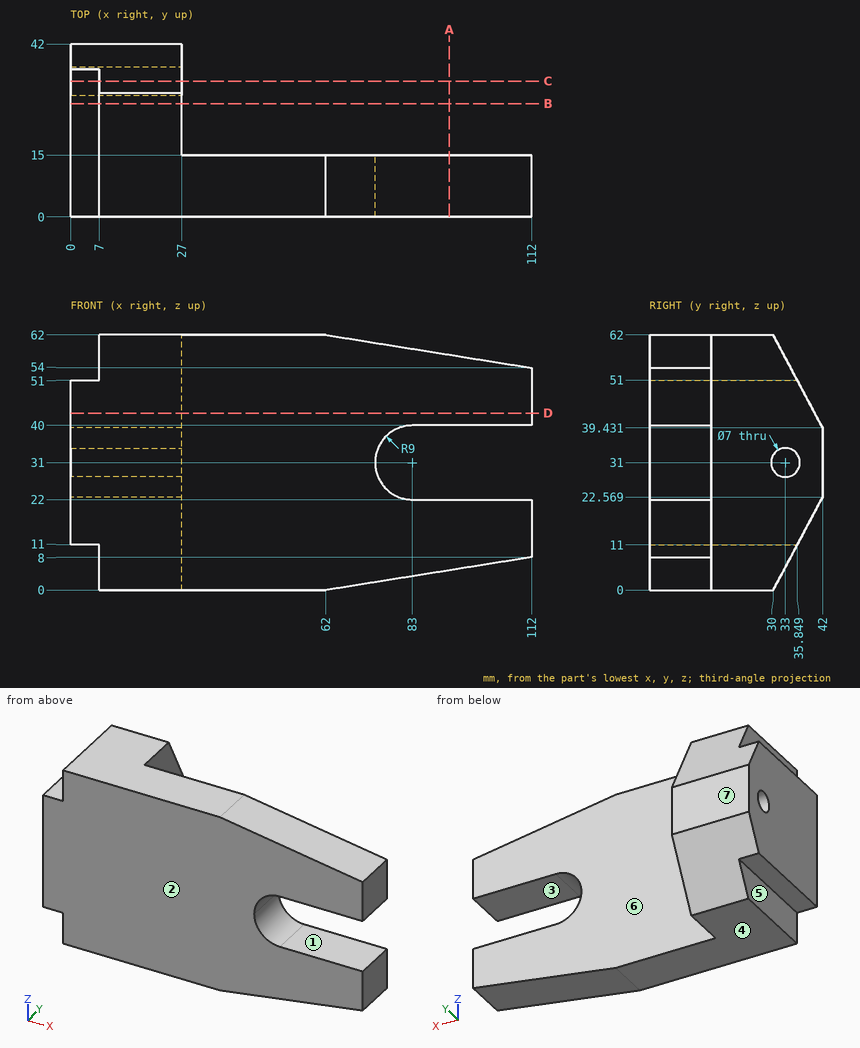
Answer from the drawing. Dimensions are ordinates in mm from the lowest x, y and z of the part. A direction names the side the tool comes from. Round coordinates to 2 decimals unless told otherwise and drop trailing zeros. Order: outer loops, then holes, each group sorted by start corner. A loop starts at its lowest first (then second) coordinate and runs counter-clockwise, first axis right, second up. Notation, with made-up numbers: (64.5, 62.25) - (71.5, 62.25) arc R18 cw to (71.5, 71.25) - close; hole circle Ø4 at (56, 55.25). An arc over 180 degrees is marked (long way). Put each result on its own line as item: value. Start each with the question number.
(1) Find section B-B (y = 27.5). Give the vertices of the cut face in (x, z), plus the area to 3 significant figures.
(2) Find section D-D (z = 43). Give the vertices of the cut face in (x, y), plus the area to 3 significant figures.
(3) Determine the mould class of the marked faces 1, 2, 3 and 4 for opening direction Z: released by +Z, released by -Z, zero draft, split by the parting line, or undercut.
(4) Given P1, Ø2, axis at x = 5, y = 15, coming from the -Z side; P2, Ø3.5, axis at x = 3, y = 20.5, coming from the +Z side; P3, Ø9, axis at y = 33, z = 31, coming from the +X side; P4, Ø10, axis at x = 81.5, z = 34.5, coming from the +Y side, each flat-ended and moving along its own axis, determine where each tip first touches the part or whether it passes through.
(5) Find section C-C (y = 33). Give the vertices of the cut face in (x, z).
(6) For the marked faces 5, 6 and 7, determine the directions among +Z, -Z, +X, -X, +Y, -Y from which every point of the face is accessible in a straight line to the end or side of a thin tool.
(7) Straight lines are drawn through the part: probe 1 along Y at (x, z) = (18.75, 31); probe 2 along X at (y, z) = (27, 17); probe 3 along Y at (x, z) = (31, 12.5). For each, find the intervals that lie inside material, in ascending order. Write a range as from..to.
(8) Find section A-A (x = 92). Give the vertices of the cut face in (y, z), plus the area to 3 significant figures.
Reply:
1. outline: (0, 11) - (7, 11) - (7, 0) - (27, 0) - (27, 62) - (7, 62) - (7, 51) - (0, 51) - close
1. area: 1,520 mm^2
2. outline: (0, 0) - (112, 0) - (112, 15) - (27, 15) - (27, 40.1) - (0, 40.1) - close
2. area: 2,360 mm^2
3. face 1: undercut
3. face 2: zero draft
3. face 3: undercut
3. face 4: released by -Z
4. P1: z = 11
4. P2: z = 51
4. P3: x = 27
4. P4: through
5. outline: (0, 11) - (7, 11) - (7, 5.64) - (27, 5.64) - (27, 27.5) - (0, 27.5) - close; (0, 34.5) - (27, 34.5) - (27, 56.36) - (7, 56.36) - (7, 51) - (0, 51) - close
6. face 5: -Z, -X, +Y, -Y
6. face 6: +Z, -Z, +X, +Y
6. face 7: +Z, -Z, +X, -X, +Y
7. probe 1: 0..29.5, 36.5..42
7. probe 2: 0..27
7. probe 3: 0..15
8. outline: (0, 4.8) - (15, 4.8) - (15, 22) - (0, 22) - close; (0, 40) - (15, 40) - (15, 57.2) - (0, 57.2) - close
8. area: 516 mm^2
